Verification items for the finished model (mm, model axes). Coordinates: 2 decimals unless noted, no trailing zeros. Loops run counter-clockwise (first coordinate to the right, second up) from the corner with the lowest first, then second, coordinate; pieces in that order, holes last. Notation, with made-up numbers: (-28.75, -14) -> (-10.75, -14) arc R8 ccw to (-10.75, 1) -> close; hole circle Ø3 at (83.25, 28.5). An arc over 180 degrees is marked (long way). Answer as a JSON object with one key per item and string values. Group by question number.
Q1. Cross-section at B-B on y = 18.5. Record the boundary of the cut face in (x, z), and give its area (3 significant figures).
Q2. Cross-section at A-A on x = 9.75. Record the boundary of the cut face in (y, z), and give its area (3 significant figures).
Q3. Cross-section at C-C on z = -12. Record the boundary of the cut face in (x, y).
Q4. Scan lines: L1, parallel to Z at x = 18.25, y = 80.5; L2, parallel to X at y = 190, z = -14.25; L3, parallel to Z at x = 16.25, y = 184.5. Record each from-to range of solid material in increasing order.
Q5. Gauge pin test, flat end, axial feed: pin 1 Ø1.5 at (x, z) = (8, -15.5) entering from +Y. Record the tip position at first contact, or that the pin passes through.
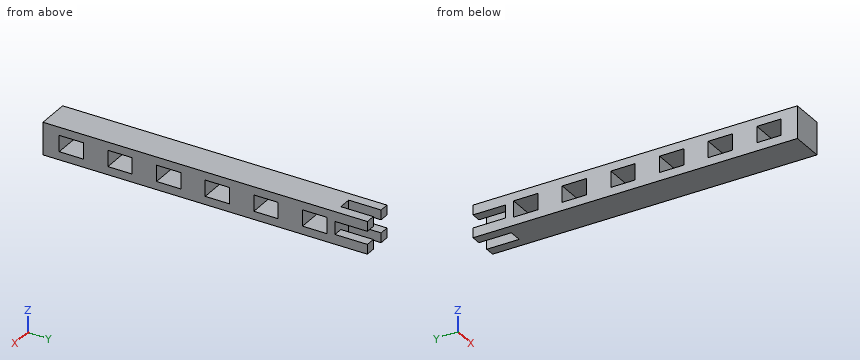
```python
from build123d import *

# Parameters (mm, degrees)
SKETCH4_W           = 20
SKETCH4_H           = 20
BOSS_EXTRUDE2_DEPTH = 200
CUT_EXTRUDE3_DEPTH  = 20
SKETCH6_W           = 10
SKETCH6_H           = 15
CUT_EXTRUDE5_DEPTH  = 21


with BuildPart() as part:
    # Sketch4 → Boss-Extrude2 (new body)
    with BuildSketch(Plane(origin=(0, 0, 0), x_dir=(1, 0, 0), z_dir=(0, 1, 0))):
        with Locations((10, 10)):
            Rectangle(SKETCH4_W, SKETCH4_H)
    extrude(amount=BOSS_EXTRUDE2_DEPTH)

    # Sketch5 → Cut-Extrude3 (cut)
    with BuildSketch(Plane(origin=(0, 200, 0), x_dir=(1, 0, 0), z_dir=(0, 1, 0))):
        Polygon((14, 20), (6, 20), (6, 14), (0, 14), (0, 6), (6, 6), (6, 0), (14, 0), (14, 6), (20, 6), (20, 14), (14, 14), align=None)
    extrude(amount=-CUT_EXTRUDE3_DEPTH, mode=Mode.SUBTRACT)

    # Sketch6 → Cut-Extrude5 (cut, through all)
    with BuildSketch(Plane(origin=(20, 0, 0), x_dir=(0, 0, -1), z_dir=(1, 0, 0))):
        with Locations((10, 17.5)):
            Rectangle(SKETCH6_W, SKETCH6_H)
        with Locations((10, 47.5)):
            Rectangle(SKETCH6_W, SKETCH6_H)
        with Locations((10, 77.5)):
            Rectangle(SKETCH6_W, SKETCH6_H)
        with Locations((10, 107.5)):
            Rectangle(SKETCH6_W, SKETCH6_H)
        with Locations((10, 137.5)):
            Rectangle(SKETCH6_W, SKETCH6_H)
        with Locations((10, 167.5)):
            Rectangle(SKETCH6_W, SKETCH6_H)
    extrude(amount=-CUT_EXTRUDE5_DEPTH, mode=Mode.SUBTRACT)


solid = part.part
```
Computed values:
{
 "1": {"outline": "(0, -20) -> (20, -20) -> (20, -15) -> (0, -15) -> close; (0, -5) -> (20, -5) -> (20, 0) -> (0, 0) -> close", "area": "200 mm²"},
 "2": {"outline": "(0, -20) -> (180, -20) -> (180, 0) -> (0, 0) -> close; hole (10, -15) -> (25, -15) -> (25, -5) -> (10, -5) -> close; hole (40, -15) -> (55, -15) -> (55, -5) -> (40, -5) -> close; hole (70, -15) -> (85, -15) -> (85, -5) -> (70, -5) -> close; hole (100, -15) -> (115, -15) -> (115, -5) -> (100, -5) -> close; hole (130, -15) -> (145, -15) -> (145, -5) -> (130, -5) -> close; hole (160, -15) -> (175, -15) -> (175, -5) -> (160, -5) -> close", "area": "2,700 mm²"},
 "3": {"outline": "(0, 0) -> (20, 0) -> (20, 10) -> (0, 10) -> close; (0, 25) -> (20, 25) -> (20, 40) -> (0, 40) -> close; (0, 55) -> (20, 55) -> (20, 70) -> (0, 70) -> close; (0, 85) -> (20, 85) -> (20, 100) -> (0, 100) -> close; (0, 115) -> (20, 115) -> (20, 130) -> (0, 130) -> close; (0, 145) -> (20, 145) -> (20, 160) -> (0, 160) -> close; (0, 175) -> (20, 175) -> (20, 180) -> (0, 180) -> close"},
 "4": {"L1": "z = -20 to -15, -5 to 0", "L2": "x = 0 to 6, 14 to 20", "L3": "z = -20 to -14, -6 to 0"},
 "5": {"pin 1": "stops at y = 180"}
}
